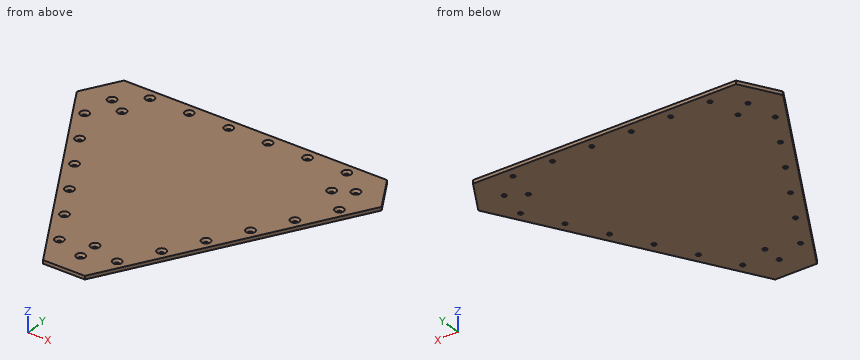
from build123d import *

# Parameters (mm, degrees)
F1_DEPTH       = 7
F3_D           = 8.8
F3_CSINK_D     = 17.92
F3_CSINK_ANGLE = 90
F5_D           = 8.8
F5_CSINK_D     = 17.92
F5_CSINK_ANGLE = 90


with BuildPart() as f1:
    # F0 (on Top) → F1 (new body)
    with BuildSketch(Plane.XY):
        Polygon((-69.6354626519, 47), (-42.5, 0), (42.5, 0), (69.6354626519, 47), (309.6354626519, 462.6921938165), (267.1354626519, 536.3043531382), (-267.1354626519, 536.3043531382), (-309.6354626519, 462.6921938165), align=None)
    extrude(amount=F1_DEPTH)

    # F3 (through all)
    with Locations(Plane.XY.offset(7)):
        with Locations((-247.682268674, 475.9982734774), (247.682268674, 475.9982734774), (0, 47)):
            CounterSinkHole(F3_D / 2, F3_CSINK_D / 2, counter_sink_angle=F3_CSINK_ANGLE)

    # F5 (through all)
    with Locations(Plane.XY.offset(7)):
        with Locations((-200, 516.3043531382), (-120, 516.3043531382), (-40, 516.3043531382), (40, 516.3043531382), (120, 516.3043531382), (200, 516.3043531382), (-258.7472232503, 414.5511776652), (-218.7472232503, 345.2691453624), (-178.7472232503, 275.9871130596), (-138.7472232503, 206.7050807569), (-98.7472232503, 137.4230484541), (-58.7472232503, 68.1410161514), (58.7472232503, 68.1410161514), (98.7472232503, 137.4230484541), (138.7472232503, 206.7050807569), (178.7472232503, 275.9871130596), (218.7472232503, 345.2691453624), (258.7472232503, 414.5511776652), (0, 87), (-213.0412525227, 455.9982734774), (213.0412525227, 455.9982734774)):
            CounterSinkHole(F5_D / 2, F5_CSINK_D / 2, counter_sink_angle=F5_CSINK_ANGLE)


solid = f1.part
Can you work these out from the model? Positions are in its coordinate system, mm. Coordinates: 2 decimals unless noted, no trailing zeros. Write each loop counter-clockwise with the first axis right and the second up, starting at its lowest first coordinate (ties: lowest second). Pieces come first, ordered by that corner, then holes. Notation, with made-up numbers: (-26, 21.5) - (15, 21.5) arc R24 ccw to (15, 36.5) - close; hole circle Ø10 at (22.25, -5.75). An arc over 180 degrees is marked (long way). Return JSON: item names as keys, results as strings. Group by question number.
Item 1: Please list where these lines run through material, in increasing order: probe 1 along Y at (x, z) = (0, 1.25); probe 2 along Y at (x, z) = (40, 1.65); probe 3 along Y at (x, z) = (120, 1.55).
Item 2: If we section it at B-B (y = 226): Write out the boundary of the cut face in (x, z), then the cut area to 3 significant figures.
Item 3: If we section it at A-A (z = 1.25): Count the separate pieces of the cut face and the enclosed holes in it, then the cut area to 3 significant figures.
Item 4: I'm going to push flat-ended pins straight in: pin 1 Ø7 at (x, y) = (178.75, 275.99) entering from +Z; pin 2 Ø10 at (x, y) = (200, 516.3) entering from +Z; pin 3 Ø4 at (y, z) = (292.5, 2) entering from +X; pin 4 Ø14 at (x, y) = (-40, 516.3) entering from +Z. Where does each tip first touch, or does it pass through?
Item 5: If we section it at C-C (y = 329): Write out the boundary of the cut face in (x, z), then the cut area to 3 significant figures.
Return value:
{
 "1": {"probe 1": "y = 0 to 42.6, 51.4 to 82.6, 91.4 to 536.3", "probe 2": "y = 0 to 511.9, 520.7 to 536.3", "probe 3": "y = 134.23 to 511.9, 520.7 to 536.3"},
 "2": {"outline": "(-172.98, 0) - (172.98, 0) - (172.98, 7) - (-172.98, 7) - close", "area": "2,420 mm^2"},
 "3": {"separate pieces": "1", "enclosed holes": "24", "area": "204,000 mm^2"},
 "4": {"pin 1": "passes through", "pin 2": "stops at z = 3.04", "pin 3": "stops at x = 212.53", "pin 4": "stops at z = 5.04"},
 "5": {"outline": "(-232.45, 0) - (232.45, 0) - (232.45, 7) - (-232.45, 7) - close", "area": "3,250 mm^2"}
}
